Autodesk Inventor part; units mm, degrees
ref_plane "YZ Plane" through (0, 0, 0) normal (1, 0, 0) x (0, 1, 0)
ref_plane "XZ Plane" through (0, 0, 0) normal (0, 1, 0) x (-1, 0, 0)
ref_plane "XY Plane" through (0, 0, 0) normal (0, 0, 1) x (1, 0, 0)
sketch "スケッチ1" plane through (0, 0, 0) normal (0, 0, 1) x (1, 0, 0)
  circle A0 centre (0, 0) radius 10.5 construction
  circle A1 centre (-13.5, 1) radius 1.35
  line L0 (-13.5, 28) -> (13.5, 28) construction
  line L1 (13.5, 28) -> (13.5, 1) construction
  line L2 (13.5, 1) -> (-13.5, 1) construction
  line L3 (-13.5, 1) -> (-13.5, 28) construction
  circle A2 centre (-13.5, 28) radius 1.35
  circle A3 centre (13.5, 1) radius 1.35
  circle A4 centre (13.5, 28) radius 1.35
  line L4 (-19.75, 10) -> (-19.75, 7.1)
  line L5 (-19.75, 10) -> (19.75, 10)
  line L6 (19.75, 10) -> (19.75, 7.1)
  line L7 (-19.75, -7.1) -> (-19.75, -10)
  line L8 (-19.75, -10) -> (19.75, -10)
  line L9 (19.75, -7.1) -> (19.75, -10)
  line L10 (-19.75, 5) -> (-21.75, 5)
  line L11 (-21.75, 5) -> (-21.75, -5)
  line L12 (-21.75, -5) -> (-19.75, -5)
  arc A5 (-19.75, 5) -> (-19.75, 7.1) centre (-19.75, 6.05) ccw
  arc A6 (-19.75, -7.1) -> (-19.75, -5) centre (-19.75, -6.05) ccw
  line L13 (19.75, 5) -> (21.75, 5)
  line L14 (21.75, 5) -> (21.75, -5)
  line L15 (21.75, -5) -> (19.75, -5)
  arc A7 (19.75, 7.1) -> (19.75, 5) centre (19.75, 6.05) ccw
  line L16 (0, 28) -> (0, 0) construction
  arc A8 (19.75, -5) -> (19.75, -7.1) centre (19.75, -6.05) ccw
  line L17 (-21.75, 0) -> (21.75, 0) construction
  circle A9 centre (0, 0) radius 6.05
  point P0 (0, 10)
  dimension "d8" = 21
  dimension "d10" = 27
  dimension "d12" = 1
  dimension "d13" = 2.7
  dimension "d38" = 27
  dimension "d44" = 27
  dimension "d47" = 1.05
  dimension "d48" = 39.5
  dimension "d49" = 2
  dimension "d50" = 10
  dimension "d51" = 5
  dimension "d52" = 12.1
extrude "押し出し1" add sketch "スケッチ1" along normal blind 2 contours L5 L6 A7 L13 L14 L15 A8 L9 L8 L7 A6 L12 L11 L10 A5 L4
sketch "スケッチ2" plane through (0, 0, 2) normal (0, 0, 1) x (1, 0, 0)
  circle A0 centre (0, 0) radius 6.05
  circle A1 centre (-13.5, 1) radius 1.35
  line L0 (-19.75, -10) -> (19.75, -10)
  line L1 (19.75, 10) -> (-19.75, 10)
  line L2 (-11.8485, 3) -> (-7.4162, 3)
  arc A2 (7.4162, 3) -> (-7.4162, 3) centre (0, 0) ccw
  line L3 (7.4162, 3) -> (11.8485, 3)
  line L4 (-18.4641, 12.448) -> (18.4641, 12.448)
  line L5 (-18.4641, 12.448) -> (-11.8485, 3)
  line L6 (11.8485, 3) -> (18.4641, 12.448)
  line L7 (-11.8485, -3) -> (-7.4162, -3)
  line L8 (-11.8485, -3) -> (-24.333, -20.8295)
  line L9 (-24.333, -20.8295) -> (24.333, -20.8295)
  line L10 (11.8485, -3) -> (7.4162, -3)
  line L11 (11.8485, -3) -> (24.333, -20.8295)
  arc A3 (-7.4162, -3) -> (7.4162, -3) centre (0, 0) ccw
  line L12 (-21.75, 5) -> (-21.75, -5)
  line L13 (-16.75, 10) -> (-19.75, 10) construction
  line L14 (0, 0) -> (-21.75, 0) construction
  line L15 (-19.75, -10) -> (-16.75, -10) construction
  line L16 (-19.75, -10) -> (19.75, -10) construction
  line L17 (0, 0) -> (0, 10) construction
  line L18 (19.75, 10) -> (16.75, 10) construction
  line L19 (19.75, -10) -> (16.75, -10) construction
  circle A4 centre (-13.5, 1) radius 2.5 construction
  dimension "d57" = 8
  dimension "d58" = 3
  dimension "d60" = 6
  dimension "d64" = 3
  dimension "d65" = 5
extrude "押し出し2" cut sketch "スケッチ2" against normal blind 10 contours L8 L7 A3 L10 L11 L0 | L0 L11 L9 L8 | L6 L3 A2 L2 L5 L1 | L1 L5 L4 L6
fillet "フィレット1" radius 2 12 edges at (-11.8485, 3, 1) (-7.4162, 3, 1) (7.4162, 3, 1) (11.8485, -3, 1) (7.4162, -3, 1) (-7.4162, -3, 1) (-11.8485, -3, 1) (-16.75, -10, 1) (-16.75, 10, 1) (16.75, 10, 1) (16.75, -10, 1) (11.8485, 3, 1)
equation "\"d38\" = d10"
equation "\"d44\" = d10"
equation "\"d50\" = d11"
equation "\"d51\" = d28"
equation "\"d60\" = 2 * d58"
equation "\"d11\" = 10"
equation "\"d28\" = 5"
properties part number "付け根_サブフレーム_1_2" material "アルミニウム 2014-T4"
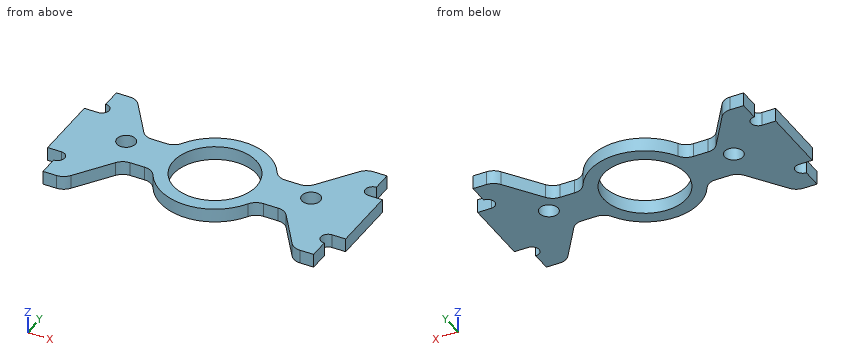
Here's how the part is built. I have some questions about the finished solid (model axes, mm). Coordinates: 2 decimals unless noted, no trailing zeros. Order: outer loops, then holes, each group sorted by start corner. A loop starts at its lowest first (then second) coordinate and runs counter-clockwise, first axis right, second up.
Item 1: If we section it at A-A on x = 0: List the corners of the cut face in (y, z) for me.
Result sheet:
outline: (-8, 0) - (-6.05, 0) - (-6.05, 2) - (-8, 2) - close; (6.05, 0) - (8, 0) - (8, 2) - (6.05, 2) - close
Item 2: If we section it at C-C on z = 1.45: State how many separate pieces and enclosed holes the cut face has, plus the area to 3 significant figures.
Result sheet:
separate pieces: 1
enclosed holes: 3
area: 405 mm2
Item 3: If we section it at D-D on y = 1.75: List the corners of the cut face in (x, z) for me.
Result sheet:
outline: (-21.75, 0) - (-14.62, 0) - (-14.62, 2) - (-21.75, 2) - close; (-12.38, 0) - (-5.79, 0) - (-5.79, 2) - (-12.38, 2) - close; (5.79, 0) - (12.38, 0) - (12.38, 2) - (5.79, 2) - close; (14.62, 0) - (21.75, 0) - (21.75, 2) - (14.62, 2) - close
Item 4: I need wall thicknesses on line 1 (X direction, y = 3.25, z = 1.6); line 2 (X direction, y = 7, z = 1.65); line 3 (X direction, y = 0.25, z = 1.6). Which ranges of each line are inside material? Lowest first, please.
Result sheet:
line 1: x = -21.75 to -11.78, -7.69 to -5.1, 5.1 to 7.69, 11.78 to 21.75
line 2: x = -19.3 to -14.65, -3.87 to 3.87, 14.65 to 19.3
line 3: x = -21.75 to -14.62, -12.38 to -6.04, 6.04 to 12.38, 14.62 to 21.75
Item 5: If we section it at B-B on y = -8.5: List the corners of the cut face in (x, z) for me.
Result sheet:
outline: (-19.75, 0) - (-15.7, 0) - (-15.7, 2) - (-19.75, 2) - close; (15.7, 0) - (19.75, 0) - (19.75, 2) - (15.7, 2) - close
Item 6: For P1, Ø0.6, axis at x = -20.5, z = 1, coming from the -Y side; P2, Ø0.6, axis at x = 10, z = 1, coming from the +Y side; P3, Ø0.6, axis at y = 9, z = 0.5, coming from the -X side, each with a flat end and sliding along its axis, tell me the tip position at first contact or that it passes through.
Result sheet:
P1: stops at y = -5
P2: stops at y = 3
P3: stops at x = -19.75
